Model file for the job. Use its own axes, mm. A direction names the side the tool comes from. Give positions to 0.01 mm unless a question says otherwise; leave off trailing zeros. Order: outer loops, then holes, each group sorted by start corner. A loop starts at its lowest first (then second) coordinate and runs counter-clockwise, first axis right, second up. Notation, with made-up numbers: (44, -30.5) - (48, -30.5) arc R23 cw to (48, 1.5) - close; hole circle Ø11 at (76.5, 58.25). An arc over 180 degrees is marked (long way). Return JSON: item names as keys, results as strings. Group by question number.
from build123d import *

# Parameters (mm, degrees)
SALIENTE_EXTRUIR1_DEPTH = 50
CROQUIS2_R              = 2.35674785
CORTAR_EXTRUIR1_DEPTH   = 20


with BuildPart() as part:
    # Croquis1 → Saliente-Extruir1 (new body)
    with BuildSketch(Plane.XY):
        with BuildLine():
            Line((-10, 0), (-10, 5.656056356))
            ThreePointArc((-10, 5.656056356), (-8.921539569, 7.959897862), (-6.461542876, 8.607338099))
            Line((-6.461542876, 8.607338099), (-5.221744043, 9.236902282))
            Line((-5.221744043, 9.236902282), (-7.354818693, 9.236902282))
            Line((-7.354818693, 9.236902282), (-7.354818693, 11))
            Line((-7.354818693, 11), (7.354818693, 11))
            Line((7.354818693, 11), (7.354818693, 9.236902282))
            Line((7.354818693, 9.236902282), (5.221744043, 9.236902282))
            Line((5.221744043, 9.236902282), (6.461542876, 8.607338099))
            ThreePointArc((6.461542876, 8.607338099), (8.921539569, 7.959897862), (10, 5.656056356))
            Line((10, 5.656056356), (10, 0))
            Line((10, 0), (25, 0))
            Line((25, 0), (25, 20))
            Line((25, 20), (-25, 20))
            Line((-25, 20), (-25, 0))
            Line((-25, 0), (-10, 0))
        make_face()
    extrude(amount=SALIENTE_EXTRUIR1_DEPTH)

    # Croquis2 → Cortar-Extruir1 (cut)
    with BuildSketch(Plane(origin=(0, 20, 0), x_dir=(1, 0, 0), z_dir=(0, 1, 0))):
        with Locations((14.831866676, -10.889102432)):
            Circle(CROQUIS2_R)
        with Locations((14.831866676, -39.461784116)):
            Circle(CROQUIS2_R)
        with Locations((-16.904414288, -39.461784116)):
            Circle(CROQUIS2_R)
        with Locations((-16.904414288, -10.889102432)):
            Circle(CROQUIS2_R)
    extrude(amount=-CORTAR_EXTRUIR1_DEPTH, mode=Mode.SUBTRACT)


solid = part.part
(1) Slice it at D-D (x = 1). Give the cut face in (y, z).
(2) Slice it at A-A (y = 6.75). Give the cut face in (x, z), and give its area (3 significant figures).
(3) Slice it at B-B (z = 36). Give the cut face in (x, y).
(4) Pull direction Y, two halves, no side cores. Call faces 4 (the face through (-25, 10, 25)), 5 (the face through (-7.355, 10, 25)), 6 (the face through (-18, 0, 25)): released by +Y, released by -Y, zero draft, split by the parting line, or undercut.
(5) Drill centre lines: L1, parallel to X at y = 1.5, z = 27.5; L2, parallel to Z at x = 15.5, y = 17.75; L3, parallel to Y at x = -2.5, z = 3. Where is each one in solid material? Low to high.
(6) Slice it at C-C (y = 15.75). Give the cut face in (x, z).
(7) 3-axis set-ups, long thin cutter, end or side, ignore diameter. For faces 1 (the face through (6, 9.237, 25)), 2 (the face through (-5.85, 8.92, 24.65)), 3 (the face through (-17.211, 10.14, 8.552)): which of +Z, -Z, +X, -X, +Y, -Y reach the whole face in a straight line?
Result set:
{
 "1": {"outline": "(11, 0) - (20, 0) - (20, 50) - (11, 50) - close"},
 "2": {"outline": "(-25, 0) - (-9.79, 0) - (-9.79, 50) - (-25, 50) - close; (9.79, 0) - (25, 0) - (25, 50) - (9.79, 50) - close; hole circle Ø4.71 at (-16.9, 10.89); hole circle Ø4.71 at (-16.9, 39.46); hole circle Ø4.71 at (14.83, 10.89); hole circle Ø4.71 at (14.83, 39.46)", "area": "1,450 mm²"},
 "3": {"outline": "(-25, 0) - (-10, 0) - (-10, 5.66) arc R3 cw to (-6.46, 8.61) - (-5.22, 9.24) - (-7.35, 9.24) - (-7.35, 11) - (7.35, 11) - (7.35, 9.24) - (5.22, 9.24) - (6.46, 8.61) arc R3 cw to (10, 5.66) - (10, 0) - (25, 0) - (25, 20) - (-25, 20) - close"},
 "4": {"face 4": "zero draft", "face 5": "undercut", "face 6": "released by -Y"},
 "5": {"L1": "x = -25 to -10, 10 to 25", "L2": "z = 0 to 8.63, 13.15 to 37.2, 41.72 to 50", "L3": "y = 11 to 20"},
 "6": {"outline": "(-25, 0) - (25, 0) - (25, 50) - (-25, 50) - close; hole circle Ø4.71 at (-16.9, 10.89); hole circle Ø4.71 at (-16.9, 39.46); hole circle Ø4.71 at (14.83, 10.89); hole circle Ø4.71 at (14.83, 39.46)"},
 "7": {"face 1": "+Z, -Z", "face 2": "+Z, -Z, -Y", "face 3": "+Y, -Y"}
}
